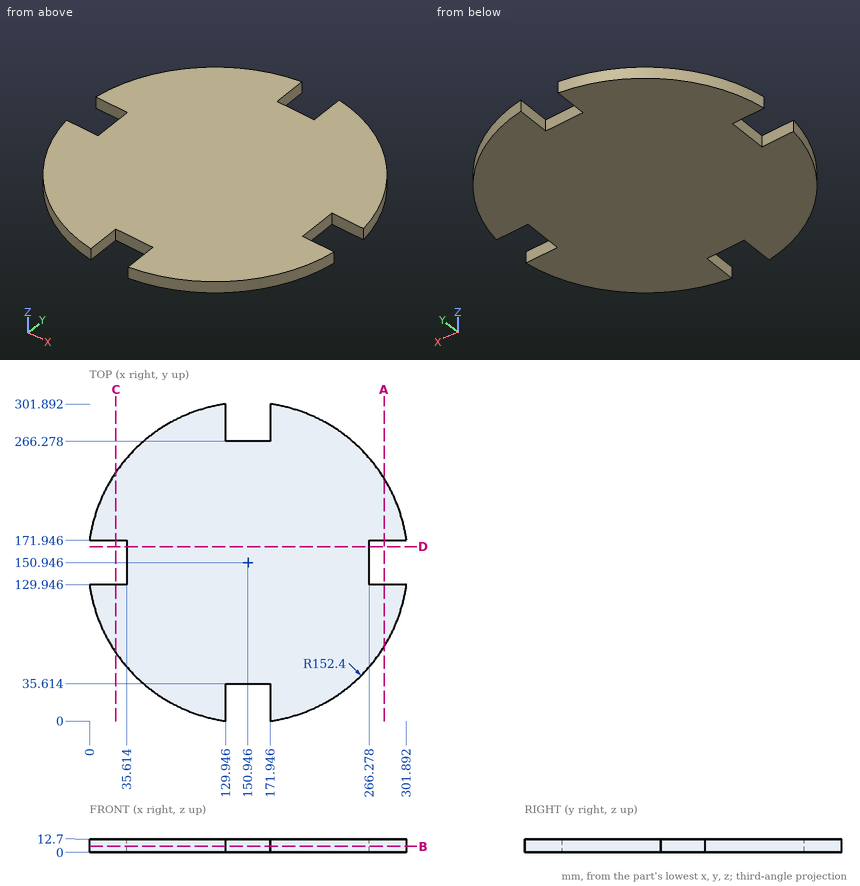
Drawing for the job (mm, zero at the part's lowest x, y, z). Coordinates: 2 decimals unless noted, no trailing zeros. Order: outer loops, then holes, each group sorted by start corner. A loop starts at its lowest first (then second) coordinate and runs counter-clockwise, first axis right, second up. Notation, with made-up numbers: (26, 18.25) -> (36, 18.25) arc R24 ccw to (36, 41.25) -> close; hole circle Ø2 at (67.5, -35.5). An arc over 180 degrees is marked (long way). Return JSON: item names as keys, results as strings.
Item 1: Pin check, flat tips, straight feed: P1, Ø6, axis at y = 213.5, z = 5.5, coming from the -X side; P2, Ø6.5, axis at x = 141.5, z = 7.5, coming from the +Y side; P3, Ø3, axis at x = 236.5, z = 6, coming from the -Y side. Stop position of each tip, or through.
Model answer:
{"P1": "stops at x = 10.66", "P2": "stops at y = 266.28", "P3": "stops at y = 23.82"}
Item 2: Slice it at A-A (x = 280.5). Write the cut outline in (y, z) (1 decimal), then the cut area to 4 significant figures.
Model answer:
{"outline": "(70.7, 0) -> (129.9, 0) -> (129.9, 12.7) -> (70.7, 12.7) -> close; (171.9, 0) -> (231.2, 0) -> (231.2, 12.7) -> (171.9, 12.7) -> close", "area": "1,505 mm²"}
Item 3: Slice it at C-C (x = 25). Write the cut outline in (y, z), then the cut area to 3 significant figures.
Model answer:
{"outline": "(65.14, 0) -> (129.95, 0) -> (129.95, 12.7) -> (65.14, 12.7) -> close; (171.95, 0) -> (236.76, 0) -> (236.76, 12.7) -> (171.95, 12.7) -> close", "area": "1,650 mm²"}
Item 4: Slice it at B-B (z = 5.75). Write the cut outline in (x, y) (1 decimal), then the cut area to 3 significant figures.
Model answer:
{"outline": "(0, 129.9) arc R152.4 ccw to (129.9, 0) -> (129.9, 35.6) -> (171.9, 35.6) -> (171.9, 0) arc R152.4 ccw to (301.9, 129.9) -> (266.3, 129.9) -> (266.3, 171.9) -> (301.9, 171.9) arc R152.4 ccw to (171.9, 301.9) -> (171.9, 266.3) -> (129.9, 266.3) -> (129.9, 301.9) arc R152.4 ccw to (0, 171.9) -> (35.6, 171.9) -> (35.6, 129.9) -> close", "area": "66,800 mm²"}
Item 5: Slice it at D-D (y = 166). Write the cut outline in (x, z) (1 decimal).
Model answer:
{"outline": "(35.6, 0) -> (266.3, 0) -> (266.3, 12.7) -> (35.6, 12.7) -> close"}
Item 6: Wall check: line 1 along Y through (x, z) = (20, 9.25) (1 decimal); line 2 along X through (y, z) = (154.5, 10.25) (1 decimal); line 3 along X through (y, z) = (177, 6). Give the ranges that are in metal, low to high. Write a range as from..to.
Model answer:
{"line 1": "y = 73..129.9, 171.9..228.9", "line 2": "x = 35.6..266.3", "line 3": "x = 0.79..301.1"}
